Here's the drawing with two shaded views (mm, measured from the low corner). I have some questions. A direction names the side the tool comes from. Give positions to 0.01 mm unless a question says otherwise; leave off trailing zeros. Order: outer loops, then holes, each group sorted by start corner. A loop starts at its lowest first (then second) coordinate and runs counter-clockwise, first axis right, second up. Notation, with made-up numbers: M -1,15 L 55,15 A10 ccw 55,28 Z; hole C 45.25,2 d5. An arc over 180 degrees is marked long. One line per question, with ' | ' between items. Start each with the question number.
1) If we section it at B-B, the plane z = 26: Please give me the cut outline in (x, y), plus the area to 3 significant figures.
2) Thinking about a two-plate mould opening in Z: for the marked faces 1, 2 and 3, which applies, +Z half, -Z half, draft (parallel to the pull), parting line (faces both ways), or undercut?
3) For the marked faces 4, 5 and 6, which set-ups out of +Z, -Z, +X, -X, +Y, -Y let a thin tool reach every point of the face, with its end or its side?
4) If we section it at A-A, the plane x = 23.25: Please give me the cut outline in (y, z), plus the area to 3 significant figures.
5) Please list where these lines run through material, in increasing order: line 1 along Z through (x, y) = (14.75, 2); line 2 along Z through (x, y) = (14, 5); line 3 along X through (y, z) = (6.75, 12.75). Write a range as [from, to].
6) I'm going to push flat-ended pins straight in: pin 1 Ø4 at (y, z) = (3, 3) entering from -X; pin 2 Ø1.5 at (x, y) = (19, 2.5) entering from +Z; pin 3 Ø1.5 at (x, y) = (18.5, 6) entering from -Z. Where does each tip first touch, or does it pass through?
7) If we section it at C-C, the plane y = 5.25: Please give me the cut outline in (x, z) (3 decimals).
8) If we section it at D-D, the plane y = 0.5: Please give me the cut outline in (x, z) (3 decimals), plus the area to 3 significant figures.
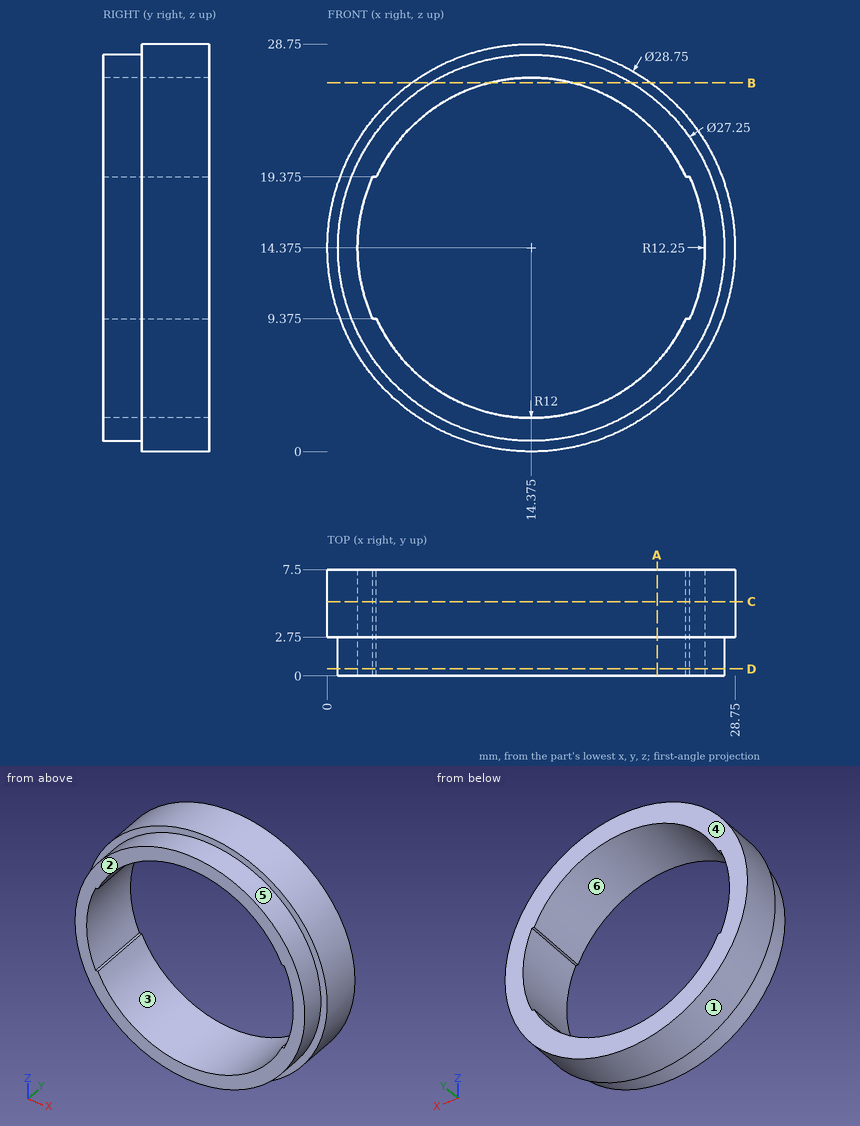
Results found:
1) outline: M 5.92,2.75 L 7.27,2.75 L 7.27,0 L 11.4,0 L 11.4,7.5 L 5.92,7.5 Z; M 17.35,0 L 21.48,0 L 21.48,2.75 L 22.83,2.75 L 22.83,7.5 L 17.35,7.5 Z | area: 74.8 mm²
2) face 1: parting line | face 2: draft | face 3: undercut
3) face 4: +Z, -Z, +X, -X, +Y | face 5: -Y | face 6: +Y, -Y
4) outline: M 0,4.04 L 2.75,4.04 L 2.75,3.07 L 7.5,3.07 L 7.5,6.3 L 0,6.3 Z; M 0,22.45 L 7.5,22.45 L 7.5,25.68 L 2.75,25.68 L 2.75,24.71 L 0,24.71 Z | area: 43.1 mm²
5) line 1: z = [0.76, 2.38], [26.37, 27.99] | line 2: z = [0, 2.38], [26.37, 28.75] | line 3: x = [0.09, 2.23], [26.52, 28.66]
6) pin 1: stops at x = 3.48 | pin 2: stops at z = 28.21 | pin 3: stops at z = 0.4
7) outline: C 14.375,14.375 d28.75; hole M 3.192,9.375 L 3.466,9.375 A12 ccw 25.284,9.375 L 25.558,9.375 A12.25 ccw 25.558,19.375 L 25.284,19.375 A12 ccw 3.466,19.375 L 3.192,19.375 A12.25 ccw Z
8) outline: C 14.375,14.375 d27.25; hole M 3.192,9.375 L 3.466,9.375 A12 ccw 25.284,9.375 L 25.558,9.375 A12.25 ccw 25.558,19.375 L 25.284,19.375 A12 ccw 3.466,19.375 L 3.192,19.375 A12.25 ccw Z | area: 126 mm²
